```python
from build123d import *

# Parameters (mm, degrees)
SKETCH_1_R          = 10
EXTRUDE_1_DEPTH     = 15
SKETCH_2_R          = 20
CUT_EXTRUDE_1_DEPTH = 13


with BuildPart() as part:
    # Эскиз1 → Бобышка-Вытянуть1 (new body, symmetric)
    with BuildSketch(Plane.XY):
        with BuildLine():
            Line((-346.502827781, 179.672535461), (11.721933855, 27.615145604))
            ThreePointArc((11.721933855, 27.615145604), (29.397741139, -5.981038033), (0, -30))
            Line((0, -30), (-546, -30))
            ThreePointArc((-546, -30), (-574.279244733, -10.014205777), (-564.879611731, 23.314378844))
            Line((-564.879611731, 23.314378844), (-377.104373367, 175.371768701))
            ThreePointArc((-377.104373367, 175.371768701), (-362.399954664, 181.765431919), (-346.502827781, 179.672535461))
        make_face()
        with Locations((-546, 0)):
            Circle(SKETCH_1_R, mode=Mode.SUBTRACT)
        with Locations((-358.224761635, 152.057389857)):
            Circle(SKETCH_1_R, mode=Mode.SUBTRACT)
        Circle(SKETCH_1_R, mode=Mode.SUBTRACT)
    extrude(amount=EXTRUDE_1_DEPTH, both=True)

    # Эскиз2 → Вырез-Вытянуть1 (cut)
    with BuildSketch(Plane(origin=(0, 0, -15), x_dir=(-1, 0, 0), z_dir=(0, 0, -1))):
        with Locations((358.224761635, 152.057389857)):
            Circle(SKETCH_2_R)
    extrude(amount=-CUT_EXTRUDE_1_DEPTH, mode=Mode.SUBTRACT)


solid = part.part
```
Verification items for the finished model (mm, model axes). A direction names the side the tool comes from. Give positions to 0.01 mm unless a question says otherwise; leave off trailing zeros. Order: outer loops, then holes, each group sorted by start corner. A loop starts at its lowest first (then second) coordinate and runs counter-clockwise, first axis right, second up. Notation, with made-up numbers: (10, -10.75) - (52, -10.75) arc R20 cw to (52, -6.75) - close; hole circle Ø3 at (16, -21). An arc over 180 degrees is marked (long way). Answer as CSV lines item,"result". Start each with the question number.
Item 1: Section check C-C, the plane x = -483. Record the boundary of the cut face in (y, z).
Item 2: Mould release check, pull along Y, two halves, no side actions. Record for faces 3 (the face through (-472.306, 98.279, 0.21)), 4 (the face through (-269, 54, -15)), 5 (the face through (-348.7, 155.1, 6.4)): released by +Y, released by -Y, zero draft, split by the parting line, or undercut.
Item 3: Gauge pin test, flat ends, axial feed: pin 1 (12 mm diameter, centred on x = -546, y = 0, fed in from +Z); pin 2 (12 mm diameter, centred on x = -366.5, y = 149.5, fed in from -Z); pin 3 (6 mm diameter, centred on x = -191.5, z = -0.5, fed in from +Y); pin 4 (8 mm diameter, centred on x = -72.5, z = 9.5, fed in from +Y). Record the tip position at first contact, or that the pin passes through.
Item 4: Material ranges on L1, parallel to Y at x = -546, z = -4; L2, parallel to X at y = 152.5, z = 11; L3, parallel to Y at x = -3, z = -2.5, recorded low to high.
Item 5: Section check B-B, the plane y = 109. Record the boundary of the cut face in (x, z).
Item 6: Access from +Z, -Z, +X, -X, +Y, -Y to the whole of each face (thin tool, end or side, straight path). Record for faces 1 (the face through (-362.625, 181.733, 0.21)), 2 (the face through (-338.244, 152.937, -8.591)).
Item 7: Section check A-A, the plane z = 9. Record the boundary of the cut face in (x, y).
Filled in:
1,outline,"(-30, -15) - (89.62, -15) - (89.62, 15) - (-30, 15) - close"
2,face 3,"released by +Y"
2,face 4,"zero draft"
2,face 5,"undercut"
3,pin 1,"through"
3,pin 2,"z = -2"
3,pin 3,"y = 115.15"
3,pin 4,"y = 65.06"
4,L1,"-30 to -10, 10 to 38.6"
4,L2,"-405.35 to -368.21, -348.23 to -282.49"
4,L3,"-30 to -9.54, 9.54 to 33.86"
5,outline,"(-459.07, -15) - (-180.01, -15) - (-180.01, 15) - (-459.07, 15) - close"
6,face 1,"+Z, -Z, +Y"
6,face 2,"-Z"
7,outline,"(-564.88, 23.31) arc R30 ccw to (-546, -30) - (0, -30) arc R30 ccw to (11.72, 27.62) - (-346.5, 179.67) arc R30 ccw to (-377.1, 175.37) - close; hole circle Ø20 at (-546, 0); hole circle Ø20 at (-358.22, 152.06); hole circle Ø20 at (0, 0)"
